```python
from build123d import *

# Parameters (mm, degrees)
SKETCH1_W           = 20.368459162
SKETCH1_H           = 6.9
SKETCH1_W_2         = 10.4
SKETCH1_H_2         = 6.8
BOSS_EXTRUDE1_DEPTH = 6


with BuildPart() as part:
    # Sketch1 → Boss-Extrude1 (new body)
    with BuildSketch(Plane.XY):
        Polygon((-451.41165464, -88.013150874), (-507.41165464, -88.013150874), (-507.41165464, -120.474064779), (-510.41165464, -123.474064779), (-510.41165464, -132.452236968), (-507.41165464, -135.452236968), (-507.41165464, -167.913150874), (-451.41165464, -167.913150874), align=None)
        with Locations((-471.27842313, -143.263150874)):
            Rectangle(SKETCH1_W, SKETCH1_H, mode=Mode.SUBTRACT)
        Polygon((-498.31165464, -127.963150874), (-498.451358752, -126.901992789), (-498.860950485, -125.913150874), (-499.512516837, -125.064013071), (-500.36165464, -124.412446718), (-501.350496555, -124.002854986), (-502.41165464, -123.863150874), (-503.472812725, -124.002854986), (-504.46165464, -124.412446718), (-505.310792443, -125.064013071), (-505.962358796, -125.913150874), (-506.371950528, -126.901992789), (-506.51165464, -127.963150874), (-506.371950528, -129.024308959), (-505.962358796, -130.013150874), (-505.310792443, -130.862288677), (-504.46165464, -131.513855029), (-503.472812725, -131.923446762), (-502.41165464, -132.063150874), (-501.350496555, -131.923446762), (-500.36165464, -131.513855029), (-499.512516837, -130.862288677), (-498.860950485, -130.013150874), (-498.451358752, -129.024308959), align=None, mode=Mode.SUBTRACT)
        Polygon((-499.970500367, -110.613150874), (-500.150321127, -111.047276593), (-500.21165464, -111.513150874), (-500.150321127, -111.979025155), (-499.970500367, -112.413150874), (-499.684446846, -112.78594308), (-499.31165464, -113.071996601), (-498.877528921, -113.251817361), (-498.41165464, -113.313150874), (-497.945780359, -113.251817361), (-497.51165464, -113.071996601), (-497.138862434, -112.78594308), (-496.852808913, -112.413150874), (-496.672988153, -111.979025155), (-496.61165464, -111.513150874), (-496.672988153, -111.047276593), (-496.852808913, -110.613150874), (-497.138862434, -110.240358668), (-497.51165464, -109.954305147), (-497.945780359, -109.774484386), (-498.41165464, -109.713150874), (-498.877528921, -109.774484386), (-499.31165464, -109.954305147), (-499.684446846, -110.240358668), align=None, mode=Mode.SUBTRACT)
        Polygon((-458.160214968, -105.890394107), (-457.990055534, -106.328396861), (-457.712330687, -106.707434531), (-457.345966918, -107.001676326), (-456.91593131, -107.191070154), (-456.451530081, -107.262709139), (-455.984411407, -107.211711202), (-455.546408653, -107.041551767), (-455.167370983, -106.763826921), (-454.873129188, -106.397463151), (-454.68373536, -105.967427544), (-454.612096375, -105.503026315), (-454.663094312, -105.035907641), (-454.833253746, -104.597904886), (-455.110978593, -104.218867216), (-455.477342363, -103.924625421), (-455.90737797, -103.735231593), (-456.371779199, -103.663592609), (-456.838897873, -103.714590546), (-457.276900628, -103.88474998), (-457.655938298, -104.162474827), (-457.950180093, -104.528838596), (-458.139573921, -104.958874204), (-458.211212905, -105.423275433), align=None, mode=Mode.SUBTRACT)
        with Locations((-493.41165464, -157.913150874)):
            Rectangle(SKETCH1_W_2, SKETCH1_H_2, mode=Mode.SUBTRACT)
        with Locations((-493.41165464, -98.013150874)):
            Rectangle(SKETCH1_W_2, SKETCH1_H_2, mode=Mode.SUBTRACT)
        with Locations((-471.27842313, -112.663150874)):
            Rectangle(SKETCH1_W, SKETCH1_H, mode=Mode.SUBTRACT)
        Polygon((-455.546408653, -148.88474998), (-455.984411407, -148.714590546), (-456.451530081, -148.663592609), (-456.91593131, -148.735231593), (-457.345966918, -148.924625421), (-457.712330687, -149.218867216), (-457.990055534, -149.597904886), (-458.160214968, -150.035907641), (-458.211212905, -150.503026315), (-458.139573921, -150.967427544), (-457.950180093, -151.397463151), (-457.655938298, -151.763826921), (-457.276900628, -152.041551767), (-456.838897873, -152.211711202), (-456.371779199, -152.262709139), (-455.90737797, -152.191070154), (-455.477342363, -152.001676326), (-455.110978593, -151.707434531), (-454.833253746, -151.328396861), (-454.663094312, -150.890394107), (-454.612096375, -150.423275433), (-454.68373536, -149.958874204), (-454.873129188, -149.528838596), (-455.167370983, -149.162474827), align=None, mode=Mode.SUBTRACT)
        with Locations((-464.41165464, -157.913150874)):
            Rectangle(SKETCH1_W_2, SKETCH1_H_2, mode=Mode.SUBTRACT)
        with Locations((-464.41165464, -98.013150874)):
            Rectangle(SKETCH1_W_2, SKETCH1_H_2, mode=Mode.SUBTRACT)
        Polygon((-499.970500367, -143.513150874), (-500.150321127, -143.947276593), (-500.21165464, -144.413150874), (-500.150321127, -144.879025155), (-499.970500367, -145.313150874), (-499.684446846, -145.68594308), (-499.31165464, -145.971996601), (-498.877528921, -146.151817361), (-498.41165464, -146.213150874), (-497.945780359, -146.151817361), (-497.51165464, -145.971996601), (-497.138862434, -145.68594308), (-496.852808913, -145.313150874), (-496.672988153, -144.879025155), (-496.61165464, -144.413150874), (-496.672988153, -143.947276593), (-496.852808913, -143.513150874), (-497.138862434, -143.140358668), (-497.51165464, -142.854305147), (-497.945780359, -142.674484386), (-498.41165464, -142.613150874), (-498.877528921, -142.674484386), (-499.31165464, -142.854305147), (-499.684446846, -143.140358668), align=None, mode=Mode.SUBTRACT)
    extrude(amount=BOSS_EXTRUDE1_DEPTH)


solid = part.part
```
Could you check a few things on this model? Use its own coordinates, in mm. A direction names the side the tool comes from. Round coordinates to 2 decimals unless told otherwise and drop trailing zeros. Loops run counter-clockwise (first coordinate to the right, second up) from the corner with the lowest first, then second, coordinate; pieces in that order, holes last. Notation, with made-up numbers: (-10.75, 49) - (44.25, 49) arc R26 cw to (44.25, 82) - close; hole circle Ø5 at (81, -27.5). An arc over 180 degrees is marked (long way). Answer as CSV lines item,"result".
1. We'd pull the mould along X, two halves only. Please class faces 1 (the face through (-481, -127, 0)), 2 (the face through (-469.612, -98, 3)), 3 (the face through (-510.412, -128, 3)), 4 (the face through (-451.412, -129, 3)): +X half, -X half, draft (parallel to the pull), parting line (faces both ways), or undercut.
Filled in:
face 1,"draft"
face 2,"undercut"
face 3,"-X half"
face 4,"+X half"
2. For pin 1 Ø1.8 at (y, z) = (-99.5, 3.5) entering from -X, with a flat end and sliding along its axis, tell me the tip position at first contact or that it passes through.
Filled in:
pin 1,"stops at x = -507.41"
3. I want a section at A-A on x = -467.5. List the corners of the cut face in (y, z) for me, then the cut area to 3 significant figures.
Filled in:
outline,"(-167.91, 0) - (-161.31, 0) - (-161.31, 6) - (-167.91, 6) - close; (-154.51, 0) - (-146.71, 0) - (-146.71, 6) - (-154.51, 6) - close; (-139.81, 0) - (-116.11, 0) - (-116.11, 6) - (-139.81, 6) - close; (-109.21, 0) - (-101.41, 0) - (-101.41, 6) - (-109.21, 6) - close; (-94.61, 0) - (-88.01, 0) - (-88.01, 6) - (-94.61, 6) - close"
area,"315 mm^2"
4. Please list where these lines run through material, in increasing order: line 1 along X through (y, z) = (-100.5, 3.9); line 2 along Y through (x, z) = (-456.5, 3.95); line 3 along Y through (x, z) = (-462.5, 5.7). Write a range as [from, to].
Filled in:
line 1,"x = [-507.41, -498.61], [-488.21, -469.61], [-459.21, -451.41]"
line 2,"y = [-167.91, -152.25], [-148.67, -107.26], [-103.68, -88.01]"
line 3,"y = [-167.91, -161.31], [-154.51, -146.71], [-139.81, -116.11], [-109.21, -101.41], [-94.61, -88.01]"
5. On a 3-axis mill with a long thin cutter (end or side, diameter ignored), from which of +Z, -Z, +X, -X, +Y, -Y can I reach the whole of each face in a straight line? I mean faces 5 (the face through (-459.212, -158, 3)), 6 (the face through (-480, -167.913, 3)), 7 (the face through (-507.412, -151, 3)). Say none if no direction works.
Filled in:
face 5,"+Z, -Z"
face 6,"+Z, -Z, +X, -X, -Y"
face 7,"+Z, -Z, -X, -Y"
6. I want a section at B-B on z = 4.65. Count the separate pieces of the cut face and the enclosed holes in it, then the cut area to 3 significant figures.
Filled in:
separate pieces,"1"
enclosed holes,"11"
area,"3,850 mm^2"
7. I want a section at C-C on y = -93. List the corners of the cut face in (x, z) for me.
Filled in:
outline,"(-507.41, 0) - (-451.41, 0) - (-451.41, 6) - (-507.41, 6) - close"
